from build123d import *

# Parameters (mm, degrees)
SKIZZE1_R                       = 5
SKIZZE1_R_2                     = 2.75
SKIZZE1_R_3                     = 2.3
SKIZZE1_W                       = 43.1
SKIZZE1_H                       = 63
AUFSATZ_LINEAR_AUSTRAGEN1_DEPTH = 10
SKIZZE3_W                       = 200
SKIZZE3_H                       = 15
AUFSATZ_LINEAR_AUSTRAGEN2_DEPTH = 150
VERRUNDUNG1_R                   = 10
AUFSATZ_LINEAR_AUSTRAGEN3_DEPTH = 10
AUFSATZ_LINEAR_AUSTRAGEN4_DEPTH = 10
VERRUNDUNG2_R                   = 10


with BuildPart() as part:
    # Skizze1 → Aufsatz-Linear austragen1 (new body)
    with BuildSketch(Plane(origin=(0, 0, 0), x_dir=(1, 0, 0), z_dir=(0, 1, 0))):
        with BuildLine():
            Line((-125, 95), (125, 95))
            ThreePointArc((125, 95), (132.071067812, 92.071067812), (135, 85))
            Line((135, 85), (135, 65))
            ThreePointArc((135, 65), (132.071067812, 57.928932188), (125, 55))
            Line((125, 55), (80, 55))
            ThreePointArc((80, 55), (69.393398282, 50.606601718), (65, 40))
            Line((65, 40), (65, -65))
            ThreePointArc((65, -65), (69.393398282, -75.606601718), (80, -80))
            Line((80, -80), (90, -80))
            Line((90, -80), (100, -80))
            Line((100, -80), (100, -95))
            Line((100, -95), (80, -95))
            Line((80, -95), (-80, -95))
            Line((-80, -95), (-100, -95))
            Line((-100, -95), (-100, -80))
            Line((-100, -80), (-90, -80))
            Line((-90, -80), (-80, -80))
            ThreePointArc((-80, -80), (-69.393398282, -75.606601718), (-65, -65))
            Line((-65, -65), (-65, 40))
            ThreePointArc((-65, 40), (-69.393398282, 50.606601718), (-80, 55))
            Line((-80, 55), (-125, 55))
            ThreePointArc((-125, 55), (-132.071067812, 57.928932188), (-135, 65))
            Line((-135, 65), (-135, 85))
            ThreePointArc((-135, 85), (-132.071067812, 92.071067812), (-125, 95))
        make_face()
        with Locations(Location((-105, 75, 0), (0, 0, 270))):
            Circle(SKIZZE1_R, mode=Mode.SUBTRACT)
        with Locations(Location((105, 75, 0), (0, 0, 90))):
            Circle(SKIZZE1_R, mode=Mode.SUBTRACT)
        with Locations(Location((-97.5, 82.5, 0), (0, 0, 270))):
            Circle(SKIZZE1_R_2, mode=Mode.SUBTRACT)
        with Locations(Location((-112.5, 67.5, 0), (0, 0, 270))):
            Circle(SKIZZE1_R_2, mode=Mode.SUBTRACT)
        with Locations(Location((97.5, 82.5, 0), (0, 0, 90))):
            Circle(SKIZZE1_R_2, mode=Mode.SUBTRACT)
        with Locations(Location((112.5, 67.5, 0), (0, 0, 90))):
            Circle(SKIZZE1_R_2, mode=Mode.SUBTRACT)
        with Locations(Location((-28.5, 53.71, 0), (0, 0, 270))):
            Circle(SKIZZE1_R_3, mode=Mode.SUBTRACT)
        with Locations(Location((-28.5, 30.71, 0), (0, 0, 90))):
            Circle(SKIZZE1_R_3, mode=Mode.SUBTRACT)
        with Locations(Location((28.5, 30.71, 0), (0, 0, 270))):
            Circle(SKIZZE1_R_3, mode=Mode.SUBTRACT)
        with Locations(Location((28.5, 53.71, 0), (0, 0, 90))):
            Circle(SKIZZE1_R_3, mode=Mode.SUBTRACT)
        with Locations((0, 42.21)):
            Rectangle(SKIZZE1_W, SKIZZE1_H, mode=Mode.SUBTRACT)
    extrude(amount=AUFSATZ_LINEAR_AUSTRAGEN1_DEPTH)

    # Skizze3 → Aufsatz-Linear austragen2 (add)
    with BuildSketch(Plane(origin=(0, 10, 0), x_dir=(1, 0, 0), z_dir=(0, 1, 0))):
        with Locations((0, -87.5)):
            Rectangle(SKIZZE3_W, SKIZZE3_H)
    extrude(amount=AUFSATZ_LINEAR_AUSTRAGEN2_DEPTH)

    # Verrundung1
    verrundung1_edges = [part.edges().sort_by_distance(p)[0] for p in [
        (-100, 160, 87.5),
        (100, 160, 87.5),
        (100, 0, 87.5),
        (-100, 0, 87.5),
    ]]
    fillet(verrundung1_edges, radius=VERRUNDUNG1_R)

    # Skizze5 → Aufsatz-Linear austragen3 (add)
    with BuildSketch(Plane.ZY.offset(50)):
        Polygon((10, 10), (80, 80), (80, 10), align=None)
    extrude(amount=-AUFSATZ_LINEAR_AUSTRAGEN3_DEPTH)

    # Skizze6 → Aufsatz-Linear austragen4 (add)
    with BuildSketch(Plane(origin=(55, 0, 0), x_dir=(0, 0, -1), z_dir=(1, 0, 0))):
        Polygon((-10, 10), (-80, 80), (-80, 10), align=None)
    extrude(amount=-AUFSATZ_LINEAR_AUSTRAGEN4_DEPTH)

    # Verrundung2
    verrundung2_edges = [part.edges().sort_by_distance(p)[0] for p in [
        (-45, 10, 10),
        (-45, 80, 80),
        (50, 10, 10),
        (50, 80, 80),
    ]]
    fillet(verrundung2_edges, radius=VERRUNDUNG2_R)


solid = part.part
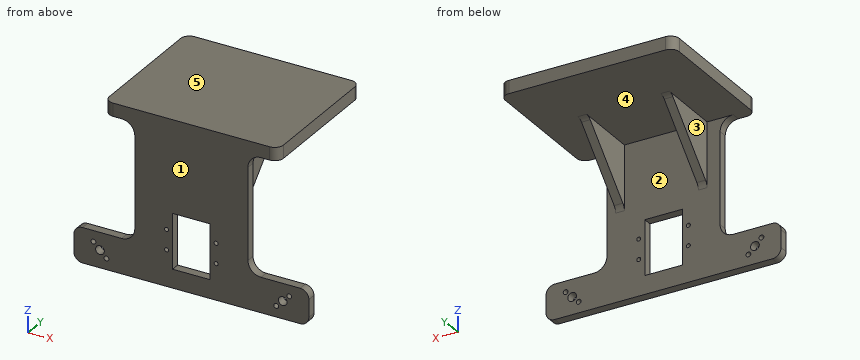
Source: CAD feature listing. Evaluate the final solid. Frame: model axes, mm. Face numbers are marked on the shaded views. A direction names the side the tool comes from. Round coordinates to 2 decimals unless told otherwise and drop trailing zeros. Order: outer loops, then holes, each group sorted by start corner. A loop starts at its lowest first (then second) coordinate and runs counter-clockwise, first axis right, second up. Notation, with made-up numbers: (-8, 50.5) -> (45, 50.5) arc R16 ccw to (45, 78.5) -> close; hole circle Ø2 at (10, -0.75). An arc over 180 degrees is marked (long way). Answer as CSV lines item,"result".
Item 1: Section B-B, the plane x = -3. Return loops of the section in (y, z), plus the area to 3 significant figures.
A:
outline,"(0, -95) -> (10, -95) -> (10, -73.71) -> (0, -73.71) -> close; (0, -10.71) -> (10, -10.71) -> (10, 80) -> (160, 80) -> (160, 95) -> (0, 95) -> close"
area,"3,520 mm²"
Item 2: Section C-C, the plane z = 60. Return loops of the section in (x, y), plus the area to 3 significant figures.
A:
outline,"(-65, 0) -> (65, 0) -> (65, 10) -> (55, 10) -> (55, 60) -> (45, 60) -> (45, 10) -> (-40, 10) -> (-40, 60) -> (-50, 60) -> (-50, 10) -> (-65, 10) -> close"
area,"2,300 mm²"
Item 3: Section A-A, the plane z = -36. Return loops of the section in (x, y).
A:
outline,"(-65, 0) -> (-21.55, 0) -> (-21.55, 10) -> (-65, 10) -> close; (21.55, 0) -> (65, 0) -> (65, 10) -> (21.55, 10) -> close"
Item 4: Line query: L1, parallel to X at y = 4, z = -82.5; L2, parallel to X at y = 7.75, z = -67.5; L3, parallel to X at y = 49, z = 54.5. Output: solid intervals per line, ascending.
A:
L1,"-135 to -100.25, -94.75 to 94.75, 100.25 to 135"
L2,"-135 to -115.25, -109.75 to -21.55, 21.55 to 109.75, 115.25 to 135"
L3,"-50 to -40, 45 to 55"
Item 5: Pin query (flat end, axial travel): pin 1 Ø3.5 at (x, z) = (-28.5, -30.71) entering from +Y; pin 2 Ø3 at (x, y) = (-113, 7) entering from +Z; pin 3 Ø7.5 at (y, z) = (61.5, 91) entering from -X; pin 4 Ø5 at (y, z) = (7, 20) entering from -X. Return the tip coordinate at first contact, or that it passes through.
A:
pin 1,"through"
pin 2,"z = -55"
pin 3,"x = -100"
pin 4,"x = -65"
Item 6: Reachability of the marked faces 1 and 2 from +Z, -Z, +X, -X, +Y, -Y: full face, straight path, thin tool, end or side. Return the list, or none.
A:
face 1,"+Z, -Z, +X, -X, -Y"
face 2,"-Z, +Y"
Item 7: Pull-direction query (X, two-part tool) for the marked faces 3, 4 and 5; classes: pulls with the +X half, pulls with the -X half, needs draft (parallel to the pull), parting line crosses it, or undercut.
A:
face 3,"pulls with the -X half"
face 4,"undercut"
face 5,"needs draft"
Item 8: Section D-D, the plane y = 126. Return loops of the section in (x, z), plus the area to 3 significant figures.
A:
outline,"(-100, 80) -> (100, 80) -> (100, 95) -> (-100, 95) -> close"
area,"3,000 mm²"
